Part print with two shaded views. Sizes in mm from the minimum x, y, z corner. A direction names the side the tool comes from. Round coordinates to 2 decimals unless told otherwise and drop trailing zeros. Write each loop counter-clockwise with the first axis right and the second up, starting at its lowest first coordinate (ties: lowest second). Pieces come first, ordered by that corner, then holes. Notation, with made-up numbers: (74.5, -18) -> (89.5, -18) arc R25 cw to (89.5, 4) -> close; hole circle Ø7 at (-7, -36.5). An arc over 180 degrees is marked (long way). Return JSON: item names as keys, results as strings.
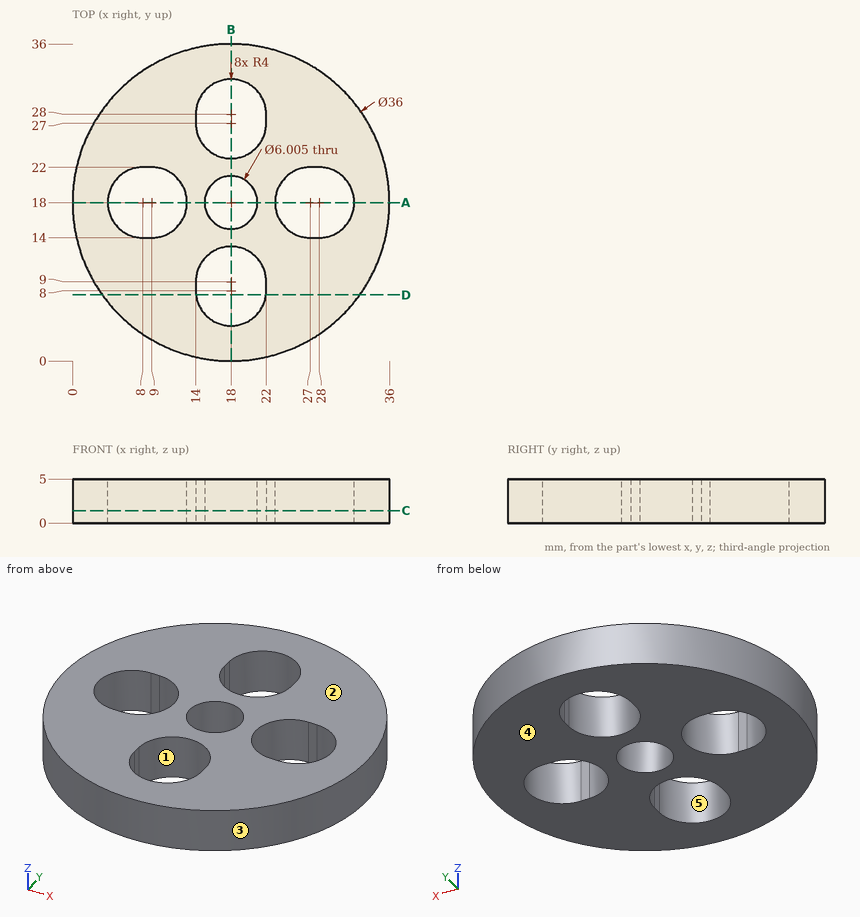
Q1. Saw through at A-A on y = 18. List the corners of the cut face in (x, z), then the cut area to 3 significant figures.
Verdict:
{"outline": "(0, 0) -> (4, 0) -> (4, 5) -> (0, 5) -> close; (13, 0) -> (15, 0) -> (15, 5) -> (13, 5) -> close; (21, 0) -> (23, 0) -> (23, 5) -> (21, 5) -> close; (32, 0) -> (36, 0) -> (36, 5) -> (32, 5) -> close", "area": "60.0 mm²"}
Q2. Saw through at D-D on y = 7.5. List the corners of the cut face in (x, z).
Verdict:
{"outline": "(3.38, 0) -> (14.03, 0) -> (14.03, 5) -> (3.38, 5) -> close; (21.97, 0) -> (32.62, 0) -> (32.62, 5) -> (21.97, 5) -> close"}
Q3. Pin check, flat tips, straight feed: pin 1 Ø0.5 at (y, z) = (27.5, 2) entering from -X; pin 2 Ø1.1 at (y, z) = (8.5, 3) entering from +X; pin 3 Ø1.5 at (y, z) = (11, 0.5) entering from +X. Stop position of each tip, or through.
Verdict:
{"pin 1": "stops at x = 2.56", "pin 2": "stops at x = 33.62", "pin 3": "stops at x = 34.88"}
Q4. 3-axis set-ups, long thin cutter, end or side, ignore diameter. For the marked faces 1 and 2: which of +Z, -Z, +X, -X, +Y, -Y reach the whole face in a straight line?
Verdict:
{"face 1": "+Z, -Z", "face 2": "+Z, +X, -X, +Y, -Y"}
Q5. Saw through at C-C on z = 1.4. List the corners of the cut face in (x, y) (1 decimal), then the cut area to 3 significant figures.
Verdict:
{"outline": "circle Ø36 at (18, 18); hole (8, 14) -> (9, 14) arc R4 ccw to (9, 22) -> (8, 22) arc R4 ccw to start; hole (14, 8) arc R4 ccw to (22, 8) -> (22, 9) arc R4 ccw to (14, 9) -> close; hole (14, 27) arc R4 ccw to (22, 27) -> (22, 28) arc R4 ccw to (14, 28) -> close; hole circle Ø6 at (18, 18); hole (27, 14) -> (28, 14) arc R4 ccw to (28, 22) -> (27, 22) arc R4 ccw to start", "area": "756 mm²"}
Q6. Wall check: L1, parallel to Y at x = 18, z = 1.9; L2, parallel to X at y = 16.5, z = 0.6. Give the ranges that are in metal, low to high.
Verdict:
{"L1": "y = 0 to 4, 13 to 15, 21 to 23, 32 to 36", "L2": "x = 0.06 to 4.29, 12.71 to 15.4, 20.6 to 23.29, 31.71 to 35.94"}
Q7. Two-plate mould, pull along X, no slides. Class the marked faces 3, 4 and 5: +X half, -X half, draft (parallel to the pull), parting line (faces both ways), or undercut.
Verdict:
{"face 3": "parting line", "face 4": "draft", "face 5": "undercut"}
